from build123d import *

# Parameters (mm, degrees)
ESBO_O1_W                = 20
ESBO_O1_H                = 15
ESBO_O1_R                = 1.5
RESSALTO_EXTRUS_O1_DEPTH = 0.5
ESBO_O2_W                = 20
ESBO_O2_H                = 2
RESSALTO_EXTRUS_O2_DEPTH = 8
CORTE_EXTRUS_O1_DEPTH    = 0.5


with BuildPart() as part:
    # Esboço1 → Ressalto-extrusão1 (new, symmetric)
    with BuildSketch(Plane.XY):
        Rectangle(ESBO_O1_W, ESBO_O1_H)
        with Locations((-8, -5.5)):
            Circle(ESBO_O1_R, mode=Mode.SUBTRACT)
        with Locations((8, -5.5)):
            Circle(ESBO_O1_R, mode=Mode.SUBTRACT)
    extrude(amount=RESSALTO_EXTRUS_O1_DEPTH, both=True)

    # Esboço2 → Ressalto-extrusão2 (add)
    with BuildSketch(Plane.XY.offset(0.5)):
        with Locations((0, 6.5)):
            Rectangle(ESBO_O2_W, ESBO_O2_H)
    extrude(amount=RESSALTO_EXTRUS_O2_DEPTH)

    # Esboço3 → Corte-extrusão1 (cut)
    # profile 1 of 6: a face of its own
    with BuildSketch(Plane(origin=(0, 0, -0.5), x_dir=(-1, 0, 0), z_dir=(0, 0, -1))):
        Polygon((-7.583333333, 3.5), (-5.878205128, 3.5), (-5.878205128, 3.141025641), (-7.269230769, 3.141025641), (-7.269230769, 2.064102564), (-5.878205128, 2.064102564), (-5.878205128, 1.705128205), (-7.269230769, 1.705128205), (-7.269230769, 0), (-7.583333333, 0), align=None)
    # profile 2 of 6: a face of its own
    with BuildSketch(Plane(origin=(0, 0, -0.5), x_dir=(-1, 0, 0), z_dir=(0, 0, -1))):
        with BuildLine():
            Line((-5.25, 3.5), (-4.549579327, 3.5))
            add(Edge.make_bspline(
                [(-4.549579327, 3.5), (-4.502838198, 3.499844414), (-4.413090054, 3.499545672), (-4.284516784, 3.497879909), (-4.167689687, 3.493105553), (-4.062669847, 3.48899697), (-3.969459192, 3.481505028), (-3.887771902, 3.474344381), (-3.817984204, 3.46497072), (-3.775738353, 3.456265297), (-3.756610577, 3.452323718)],
                knots=[0, 0, 0, 0, 1.410062039, 2.707475311, 3.878576406, 4.937260626, 5.877586885, 6.699081471, 7.410979367, 8, 8, 8, 8], degree=3))
            add(Edge.make_bspline(
                [(-3.756610577, 3.452323718), (-3.731003953, 3.445996953), (-3.680336963, 3.433478389), (-3.607386897, 3.407018788), (-3.537872573, 3.376399163), (-3.472082749, 3.340435443), (-3.410346958, 3.298860663), (-3.352028647, 3.252392541), (-3.296863184, 3.201285335), (-3.247081553, 3.144250494), (-3.200142502, 3.084413984), (-3.160553875, 3.019710227), (-3.126427396, 2.9520487), (-3.099256879, 2.880741282), (-3.077378905, 2.80647951), (-3.061952666, 2.728590713), (-3.052701478, 2.647429738), (-3.051759623, 2.59207183), (-3.051282051, 2.564002404)],
                knots=[0, 0, 0, 0, 1.027469482, 2.033020251, 3.019912614, 3.986113645, 4.951240523, 5.91722682, 6.890402269, 7.87763091, 8.8651537, 9.85103654, 10.82876324, 11.815024772, 12.821070561, 13.842952187, 14.906261191, 16, 16, 16, 16], degree=3))
            add(Edge.make_bspline(
                [(-3.051282051, 2.564002404), (-3.052751049, 2.517367299), (-3.055617445, 2.426370131), (-3.082342549, 2.29430925), (-3.126119069, 2.171119935), (-3.186442358, 2.056957297), (-3.263261833, 1.954046652), (-3.355586624, 1.863656197), (-3.463468236, 1.788016284), (-3.563897552, 1.735563479), (-3.652611752, 1.701970571), (-3.725645064, 1.678334212), (-3.805312042, 1.660072247), (-3.890849376, 1.643712115), (-3.982613032, 1.63136042), (-4.080383071, 1.622313826), (-4.184229223, 1.616659777), (-4.255568292, 1.615817772), (-4.292267628, 1.615384615)],
                knots=[0, 0, 0, 0, 1.260483769, 2.459530307, 3.627416485, 4.787058657, 5.939039949, 7.08810263, 8.267026773, 9.491475466, 10.141966685, 10.831826277, 11.566392101, 12.351337768, 13.187381173, 14.07005841, 15.007169909, 16, 16, 16, 16], degree=3))
            Line((-4.292267628, 1.615384615), (-3.006410256, 0))
            Line((-3.006410256, 0), (-3.394831731, 0))
            Line((-3.394831731, 0), (-4.680689103, 1.615384615))
            Line((-4.680689103, 1.615384615), (-4.935897436, 1.615384615))
            Line((-4.935897436, 1.615384615), (-4.935897436, 0))
            Line((-4.935897436, 0), (-5.25, 0))
            Line((-5.25, 0), (-5.25, 3.5))
        make_face()
        with BuildLine():
            Line((-4.935897436, 3.141025641), (-4.935897436, 1.974358974))
            Line((-4.935897436, 1.974358974), (-4.295072115, 1.969451122))
            add(Edge.make_bspline(
                [(-4.295072115, 1.969451122), (-4.265152076, 1.969437885), (-4.207158519, 1.969412229), (-4.123257855, 1.973406005), (-4.045137743, 1.977949323), (-3.973096991, 1.984898669), (-3.907103415, 1.99385474), (-3.847190002, 2.005057725), (-3.79325895, 2.018109787), (-3.730360412, 2.038311413), (-3.66012388, 2.070317431), (-3.583792421, 2.11688293), (-3.518790083, 2.175452049), (-3.463872221, 2.242425505), (-3.419742789, 2.316061754), (-3.388630735, 2.395478123), (-3.368888292, 2.478669721), (-3.366559747, 2.535847829), (-3.365384615, 2.564703526)],
                knots=[0, 0, 0, 0, 1.146690395, 2.22261258, 3.21895312, 4.145990853, 4.996080663, 5.770904154, 6.481378293, 7.121626537, 8.300444488, 9.431385265, 10.535395872, 11.636531494, 12.74115979, 13.810798291, 14.895190096, 16, 16, 16, 16], degree=3))
            add(Edge.make_bspline(
                [(-3.365384615, 2.564703526), (-3.366586736, 2.592850099), (-3.368968902, 2.648626338), (-3.38841767, 2.730282248), (-3.421307052, 2.807349198), (-3.46562929, 2.879513683), (-3.519628445, 2.945019419), (-3.582946257, 3.001066572), (-3.653851452, 3.047316037), (-3.720122651, 3.076870418), (-3.779356863, 3.094990271), (-3.830786523, 3.107741435), (-3.888898001, 3.117985904), (-3.95397346, 3.126193964), (-4.02573509, 3.133248909), (-4.104545742, 3.138000687), (-4.189882522, 3.140814551), (-4.249029453, 3.14095364), (-4.279647436, 3.141025641)],
                knots=[0, 0, 0, 0, 1.101028733, 2.181837193, 3.264309656, 4.369019818, 5.486613113, 6.575447106, 7.666700264, 8.788928104, 9.402425223, 10.0903467, 10.862060571, 11.710948788, 12.657782767, 13.684531032, 14.801375019, 16, 16, 16, 16], degree=3))
            Line((-4.279647436, 3.141025641), (-4.935897436, 3.141025641))
        make_face(mode=Mode.SUBTRACT)
    # profile 3 of 6: a face of its own
    with BuildSketch(Plane(origin=(0, 0, -0.5), x_dir=(-1, 0, 0), z_dir=(0, 0, -1))):
        Polygon((-2.288461538, 3.5), (-0.314102564, 3.5), (-0.314102564, 3.141025641), (-1.974358974, 3.141025641), (-1.974358974, 2.064102564), (-0.314102564, 2.064102564), (-0.314102564, 1.705128205), (-1.974358974, 1.705128205), (-1.974358974, 0.358974359), (-0.314102564, 0.358974359), (-0.314102564, 0), (-2.288461538, 0), align=None)
    # profile 4 of 6: a face of its own
    with BuildSketch(Plane(origin=(0, 0, -0.5), x_dir=(-1, 0, 0), z_dir=(0, 0, -1))):
        Polygon((0.314102564, 0), (0.314102564, 3.5), (0.380008013, 3.5), (2.692307692, 0.745292468), (2.692307692, 3.5), (3.006410256, 3.5), (3.006410256, 0), (2.934895833, 0), (0.628205128, 2.748397436), (0.628205128, 0), align=None)
    # profile 5 of 6: a face of its own
    with BuildSketch(Plane(origin=(0, 0, -0.5), x_dir=(-1, 0, 0), z_dir=(0, 0, -1))):
        Polygon((3.5, 3.141025641), (3.5, 3.5), (5.33974359, 3.5), (5.33974359, 3.141025641), (4.576923077, 3.141025641), (4.576923077, 0), (4.262820513, 0), (4.262820513, 3.141025641), align=None)
    # profile 6 of 6: a face of its own
    with BuildSketch(Plane(origin=(0, 0, -0.5), x_dir=(-1, 0, 0), z_dir=(0, 0, -1))):
        Polygon((5.878205128, 3.5), (7.852564103, 3.5), (7.852564103, 3.141025641), (6.192307692, 3.141025641), (6.192307692, 2.064102564), (7.852564103, 2.064102564), (7.852564103, 1.705128205), (6.192307692, 1.705128205), (6.192307692, 0.358974359), (7.852564103, 0.358974359), (7.852564103, 0), (5.878205128, 0), align=None)
    extrude(amount=-CORTE_EXTRUS_O1_DEPTH, mode=Mode.SUBTRACT)


solid = part.part
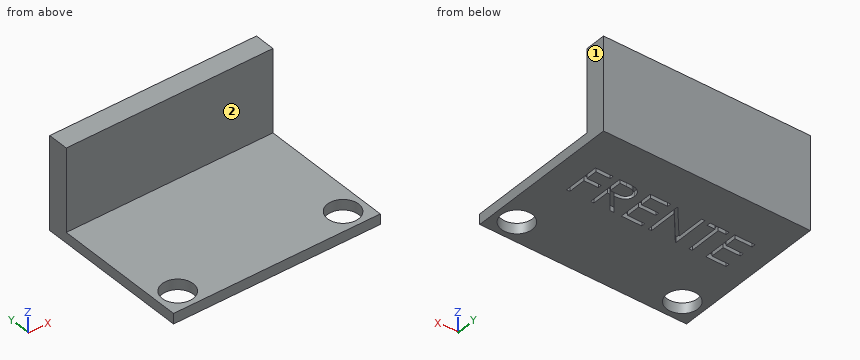
Here's how the part is built. I have some questions about the finished solid (model axes, mm). Face numbers are marked on the shaded views. A direction names the side the tool comes from. Give positions to 0.01 mm unless a question says otherwise; leave off trailing zeros. Order: outer loops, then holes, each group sorted by start corner. A loop starts at its lowest first (then second) coordinate and runs counter-clockwise, first axis right, second up. Notation, with made-up numbers: (63, 63.25) -> (75, 63.25) arc R24 ccw to (75, 76.25) -> close; hole circle Ø2 at (-29, 77). An arc over 180 degrees is marked (long way). Use a Markdown table: item, result. Add a question column.
Item 1: I need wall thicknesses on line 1 (Y direction, x = -8, z = 0.05); line 2 (Z direction, x = -3, y = 5.25); line 3 (Y direction, x = 4, z = 3.75). Which ranges of each line are inside material? Lowest first, please.
Item 2: Imagine slicing it at B-B on x = 8. Please give me the cut outline in (y, z), plus the area to 3 significant figures.
Item 3: Imagine slicing it at A-A on y = -4.25. Please give me the cut outline in (x, z), plus the area to 3 significant figures.
Item 4: For the marked faces 1 and 2, which set-ups out of +Z, -Z, +X, -X, +Y, -Y let a thin tool reach every point of the face, with its end or its side?
Item 5: Imagine slicing it at C-C on z = 2.25. Please give me the cut outline in (x, y).
Item 6: Imagine slicing it at D-D on x = -2. Please give me the cut outline in (y, z), plus the area to 3 significant figures.
Data:
| question | item | result |
|---|---|---|
| 1 | line 1 | y = -7.5 to -7, -4 to 7.5 |
| 1 | line 2 | z = -0.5 to 0.5 |
| 1 | line 3 | y = 5.5 to 7.5 |
| 2 | outline | (-7.5, -0.5) -> (-7, -0.5) -> (-7, 0.5) -> (-7.5, 0.5) -> close; (-4, -0.5) -> (7.5, -0.5) -> (7.5, 8.5) -> (5.5, 8.5) -> (5.5, 0.5) -> (-4, 0.5) -> close |
| 2 | area | 28.0 mm² |
| 3 | outline | (-10, -0.5) -> (-8.83, -0.5) -> (-8.83, 0.5) -> (-10, 0.5) -> close; (-7.17, -0.5) -> (7.17, -0.5) -> (7.17, 0.5) -> (-7.17, 0.5) -> close; (8.83, -0.5) -> (10, -0.5) -> (10, 0.5) -> (8.83, 0.5) -> close |
| 3 | area | 16.7 mm² |
| 4 | face 1 | +Z, -Z, +X, +Y, -Y |
| 4 | face 2 | +Z, +X, -X, -Y |
| 5 | outline | (-10, 5.5) -> (10, 5.5) -> (10, 7.5) -> (-10, 7.5) -> close |
| 6 | outline | (-7.5, -0.5) -> (1.11, -0.5) -> (1.11, 0) -> (1.57, 0) -> (1.57, -0.5) -> (7.5, -0.5) -> (7.5, 8.5) -> (5.5, 8.5) -> (5.5, 0.5) -> (-7.5, 0.5) -> close |
| 6 | area | 30.8 mm² |
